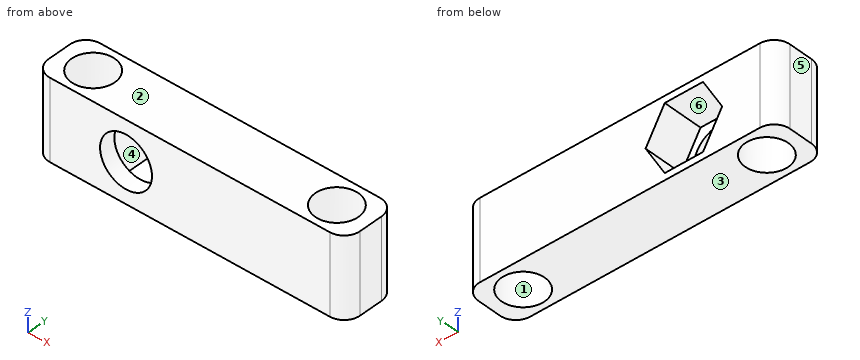
```python
from build123d import *

# Parameters (mm, degrees)
CROQUIS1_W              = 39
CROQUIS1_H              = 7
CROQUIS1_R              = 2.7
SALIENTE_EXTRUIR1_DEPTH = 10
CORTAR_EXTRUIR1_DEPTH   = 7
REDONDEO1_R             = 2
CROQUIS4_R              = 3.25
SALIENTE_EXTRUIR2_DEPTH = 2


with BuildPart() as part:
    # Croquis1 → Saliente-Extruir1 (new body)
    with BuildSketch(Plane.XY):
        with Locations((-26.516694491, 12.37804878)):
            Rectangle(CROQUIS1_W, CROQUIS1_H)
        with Locations((-41.766694491, 12.37804878)):
            Circle(CROQUIS1_R, mode=Mode.SUBTRACT)
        with Locations((-11.266694491, 12.37804878)):
            Circle(CROQUIS1_R, mode=Mode.SUBTRACT)
    extrude(amount=SALIENTE_EXTRUIR1_DEPTH)

    # Croquis2 → Cortar-Extruir1 (cut)
    with BuildSketch(Plane.XZ.offset(-8.87804878)):
        Polygon((-29.724687257, 5), (-32.120690874, 9.15), (-36.912698108, 9.15), (-39.308701725, 5), (-36.912698108, 0.85), (-32.120690874, 0.85), align=None)
    extrude(amount=-CORTAR_EXTRUIR1_DEPTH, mode=Mode.SUBTRACT)

    # Redondeo1
    redondeo1_edges = [part.edges().sort_by_distance(p)[0] for p in [
        (-46.016694491, 15.87804878, 5),
        (-7.016694491, 15.87804878, 5),
        (-7.016694491, 8.87804878, 5),
        (-46.016694491, 8.87804878, 5),
    ]]
    fillet(redondeo1_edges, radius=REDONDEO1_R)

    # Croquis4 → Saliente-Extruir2 (add)
    with BuildSketch(Plane.XZ.offset(-8.87804878)):
        Polygon((-29.724687257, 5), (-32.120690874, 9.15), (-36.912698108, 9.15), (-39.308701725, 5), (-36.912698108, 0.85), (-32.120690874, 0.85), align=None)
        with Locations(Location((-34.516694491, 5, 0), (0, 0, 270))):
            Circle(CROQUIS4_R, mode=Mode.SUBTRACT)
    extrude(amount=-SALIENTE_EXTRUIR2_DEPTH)


solid = part.part
```
Check sheet for the modelled part. Datum: model origin and axes. Units: mm. Face numbers are marked on the shaded views. A direction names the side the tool comes from. Round coordinates to 2 decimals unless told otherwise and drop trailing zeros. Order: outer loops, then holes, each group sorted by start corner. A loop starts at its lowest first (then second) coordinate and runs counter-clockwise, first axis right, second up. Notation, with made-up numbers: (71, 54) - (103, 54) arc R20 cw to (103, 69) - close; hole circle Ø6 at (67.25, 75.5). An arc over 180 degrees is marked (long way). Answer as CSV lines item,"result". Start each with the question number.
1) Tool access check on the marked faces 5 and 6. Record the directions out of +Z, -Z, +X, -X, +Y, -Y that give a thin tool (end or side, any length) a straight path to the whole face; none if there is none.
2) Section check B-B (z = 1.25). Record the cut outline in (x, y), then the cut area to 3 significant figures.
3) Scan lines: probe 1 along X at (y, z) = (13.5, 8.5); probe 2 along X at (y, z) = (12.75, 2.75); probe 3 along X at (y, z) = (10.75, 9.5). Record each from-to range of solid material in increasing order.
4) Section check A-A (x = -13.5). Record the cut outline in (y, z), then the cut area to 3 significant figures.
5) Depth check by flat-ended pin: pin 1 (4 mm diameter, centred on x = -34.52, z = 5, fed in from +Y); pin 2 (2.5 mm diameter, centred on x = -35.5, z = 7, fed in from +Y). Enter the tip coordinate at first touch or a pass-through.
6) Draft check along Z on the marked faces 1, 2, 3 and 4. Enter one of: +Z half, -Z half, draft (parallel to the pull), parting line (faces both ways), or undercut.
Determined:
1,face 5,"+Z, -Z, -X, +Y, -Y"
1,face 6,"+Y"
2,outline,"(-46.02, 10.88) arc R2 ccw to (-44.02, 8.88) - (-9.02, 8.88) arc R2 ccw to (-7.02, 10.88) - (-7.02, 13.88) arc R2 ccw to (-9.02, 15.88) - (-31.89, 15.88) - (-31.89, 10.88) - (-37.14, 10.88) - (-37.14, 15.88) - (-44.02, 15.88) arc R2 ccw to (-46.02, 13.88) - close; hole circle Ø5.4 at (-41.77, 12.38); hole circle Ø5.4 at (-11.27, 12.38)"
2,area,"197 mm^2"
3,probe 1,"-46.02 to -44.22, -39.31 to -37.29, -31.75 to -13.72, -8.81 to -7.02"
3,probe 2,"-46.02 to -44.44, -39.09 to -38.01, -31.02 to -13.94, -8.59 to -7.02"
3,probe 3,"-46.01 to -43.92, -39.61 to -13.42, -9.11 to -7.02"
4,outline,"(8.88, 0) - (10.86, 0) - (10.86, 10) - (8.88, 10) - close; (13.9, 0) - (15.88, 0) - (15.88, 10) - (13.9, 10) - close"
4,area,"39.7 mm^2"
5,pin 1,"through"
5,pin 2,"y = 10.88"
6,face 1,"draft"
6,face 2,"+Z half"
6,face 3,"-Z half"
6,face 4,"undercut"
